```python
from build123d import *

# Parameters (mm, degrees)
SKETCH1_W           = 50
SKETCH1_H           = 20
BOSS_EXTRUDE1_DEPTH = 6
SKETCH2_W           = 6
SKETCH2_H           = 20
BOSS_EXTRUDE2_DEPTH = 44
SKETCH3_W           = 44
SKETCH3_H           = 6
BOSS_EXTRUDE3_DEPTH = 44
SKETCH5_R           = 1.25
CUT_EXTRUDE1_DEPTH  = 74.484692283


with BuildPart() as part:
    # Sketch1 → Boss-Extrude1 (new body)
    with BuildSketch(Plane(origin=(0, 0, 0), x_dir=(1, 0, 0), z_dir=(0, 1, 0))):
        with Locations((25, 10)):
            Rectangle(SKETCH1_W, SKETCH1_H)
    extrude(amount=BOSS_EXTRUDE1_DEPTH)

    # Sketch2 → Boss-Extrude2 (add)
    with BuildSketch(Plane(origin=(0, 6, 0), x_dir=(1, 0, 0), z_dir=(0, 1, 0))):
        with Locations((47, 10)):
            Rectangle(SKETCH2_W, SKETCH2_H)
    extrude(amount=BOSS_EXTRUDE2_DEPTH)

    # Sketch3 → Boss-Extrude3 (add)
    with BuildSketch(Plane(origin=(0, 6, 0), x_dir=(1, 0, 0), z_dir=(0, 1, 0))):
        with Locations((22, 3)):
            Rectangle(SKETCH3_W, SKETCH3_H)
    extrude(amount=BOSS_EXTRUDE3_DEPTH)

    # Sketch5 → Cut-Extrude1 (cut, through all)
    with BuildSketch(Plane.XY):
        with Locations((6, 44)):
            Circle(SKETCH5_R)
        with Locations((38, 44)):
            Circle(SKETCH5_R)
        with Locations((5.302448234, 12)):
            Circle(SKETCH5_R)
        with Locations((37.302448234, 12)):
            Circle(SKETCH5_R)
    extrude(amount=-CUT_EXTRUDE1_DEPTH, mode=Mode.SUBTRACT)


solid = part.part
```
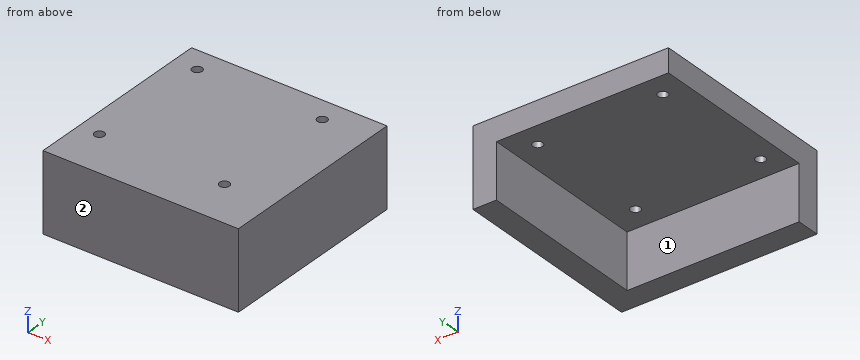
Design review of the part built by this model. Coordinates are the model's own, in mm. Face numbers are marked on the shaded views. A direction names the side the tool comes from. Coordinates: 2 decimals unless noted, no trailing zeros. Order: outer loops, then holes, each group sorted by start corner. A loop starts at its lowest first (then second) coordinate and runs counter-clockwise, first axis right, second up.
1) Take a section at C-C, the plane z = -13.5. Give the boundary of the cut face in (x, y).
2) Take a section at B-B, the plane x = 19.5. Give the boundary of the cut face in (y, z).
3) Wall thickness on line 1 along Y through (x, z) = (6, -2.55); line 2 along Z through (x, y) = (13, 19); line 3 along Y through (x, z) = (25, -9.75): over which ranges is each line inside the solid? List them lowest first.
4) For the marked faces 1 and 2, list the 3-axis set-ups (+Z, -Z, +X, -X, +Y, -Y) from which the entire face can be reached by the end or side of a thin tool; tool diameter is ignored.
5) Take a section at A-A, the plane y = 12. Give the boundary of the cut face in (x, z), and give its area (3 significant figures).
6) Clearance check with flat-ended pins moving along their axes: pin 1 (8 mm diameter, centred on x = 16.5, y = 39.5, fed in from -Z); pin 2 (7 mm diameter, centred on y = 23.5, z = -16, fed in from -X); pin 3 (1.5 mm diameter, centred on x = 37.3, y = 12, fed in from -Z). State where each tip first meets the part, or that it passes through.
Returned:
1. outline: (0, 0) - (50, 0) - (50, 50) - (44, 50) - (44, 6) - (0, 6) - close
2. outline: (0, -20) - (6, -20) - (6, -6) - (50, -6) - (50, 0) - (0, 0) - close
3. line 1: y = 0 to 10.96, 13.04 to 42.75, 45.25 to 50
3. line 2: z = -6 to 0
3. line 3: y = 0 to 6
4. face 1: -Z, -X, +Y
4. face 2: +Z, -Z, +X, -X, -Y
5. outline: (0, -6) - (4.05, -6) - (4.05, 0) - (0, 0) - close; (6.55, -6) - (36.05, -6) - (36.05, 0) - (6.55, 0) - close; (38.55, -6) - (44, -6) - (44, -20) - (50, -20) - (50, 0) - (38.55, 0) - close
5. area: 354 mm2
6. pin 1: stops at z = -6
6. pin 2: stops at x = 44
6. pin 3: passes through
